from build123d import *

# Parameters (mm, degrees)
F0_W     = 78
F0_H     = 158.5
F0_R     = 5.75
F0_R_2   = 0.75
F0_W_2   = 14
F0_H_2   = 1
F0_W_3   = 22
F0_H_3   = 12
F1_DEPTH = 7
F2_R     = 3.49999


# Not quite as in the source:
# - a fillet or chamfer is up to 0.001 mm smaller than in the source, because OpenCascade refuses the exact size


with BuildPart() as f1:
    # F0 (on Top) → F1 (new body)
    with BuildSketch(Plane.XY):
        Rectangle(F0_W, F0_H)
        with Locations((0, -69.5)):
            Circle(F0_R, mode=Mode.SUBTRACT)
        with Locations((-13.75, 69.75)):
            Circle(F0_R_2, mode=Mode.SUBTRACT)
        with Locations((0, 69.75)):
            Rectangle(F0_W_2, F0_H_2, mode=Mode.SUBTRACT)
        with Locations((22.5, 67.75)):
            Rectangle(F0_W_3, F0_H_3, mode=Mode.SUBTRACT)
        with Locations((0, -69.5)):
            Circle(F0_R)
        with Locations((22.5, 67.75)):
            Rectangle(F0_W_3, F0_H_3)
        with Locations((0, 69.75)):
            Rectangle(F0_W_2, F0_H_2)
        with Locations((-13.75, 69.75)):
            Circle(F0_R_2)
    extrude(amount=F1_DEPTH)

    # F2 (radius 3.5 in the source; OpenCascade refuses exactly that, so slightly less here)
    f2_edges = [f1.edges().sort_by_distance(p)[0] for p in [
        (39, 0, 7),
        (-39, 0, 7),
        (0, -79.25, 7),
        (0, 79.25, 7),
        (39, 0, 0),
        (0, -79.25, 0),
        (0, 79.25, 0),
        (-39, 0, 0),
        (-39, 79.25, 3.5),
        (39, 79.25, 3.5),
        (-39, -79.25, 3.5),
        (39, -79.25, 3.5),
    ]]
    fillet(f2_edges, radius=F2_R)


solid = f1.part
Could you check a few things on this model? Use its own coordinates, in mm. Give positions to 0.01 mm unless a question says otherwise; leave off trailing zeros. Loops run counter-clockwise (first coordinate to the right, second up) from the corner with the lowest first, then second, coordinate; pieces in that order, holes last. Notation, with made-up numbers: (15, 30) -> (46, 30) arc R17 cw to (46, 61) -> close; hole circle Ø3 at (18, 37). An arc over 180 degrees is marked (long way). Return JSON: item names as keys, results as strings.
Item 1: I need wall thicknesses on L1, parallel to X at y = -32, z = 3.25; L2, parallel to Z at x = 36, y = -15.5; L3, parallel to X at y = 43.5, z = 1.75. Which ranges of each line are inside material? Lowest first, please. Write a range as from..to.
Geometry results:
{"L1": "x = -38.99..38.99", "L2": "z = 0.04..6.96", "L3": "x = -38.53..38.53"}
Item 2: If we section it at B-B on z = 1.75: List the corners of the cut face in (x, y) for me, plus the area to 3 significant figures.
Geometry results:
{"outline": "(-38.53, -75.75) arc R3.03 ccw to (-35.5, -78.78) -> (35.5, -78.78) arc R3.03 ccw to (38.53, -75.75) -> (38.53, 75.75) arc R3.03 ccw to (35.5, 78.78) -> (-35.5, 78.78) arc R3.03 ccw to (-38.53, 75.75) -> close", "area": "12,100 mm²"}
Item 3: I'm going to push a flat-ended pin straight in: pin 1 (3 mm diameter, centred on y = 42, z = 0.5, fed in from +X). Where does the tip first touch, or does it pass through?
Geometry results:
{"pin 1": "stops at x = 38.66"}
